Source: three-view drawing plus pictorial views. Frame: mm from the lowest corner of the part. A direction names the side the tool comes from. Give positions to 0.01 mm unless a question says otherwise; leave off trailing zeros. Order: outer loops, then holes, each group sorted by start corner. A loop starts at its lowest first (then second) coordinate and runs counter-clockwise, first axis right, second up. Notation, with made-up numbers: (-20.75, 38.25) -> (19.25, 38.25) arc R16 cw to (19.25, 65.25) -> close; hole circle Ø9 at (74.25, 35). An arc over 180 degrees is marked (long way). Use a Markdown table: item, result. Add a question column.
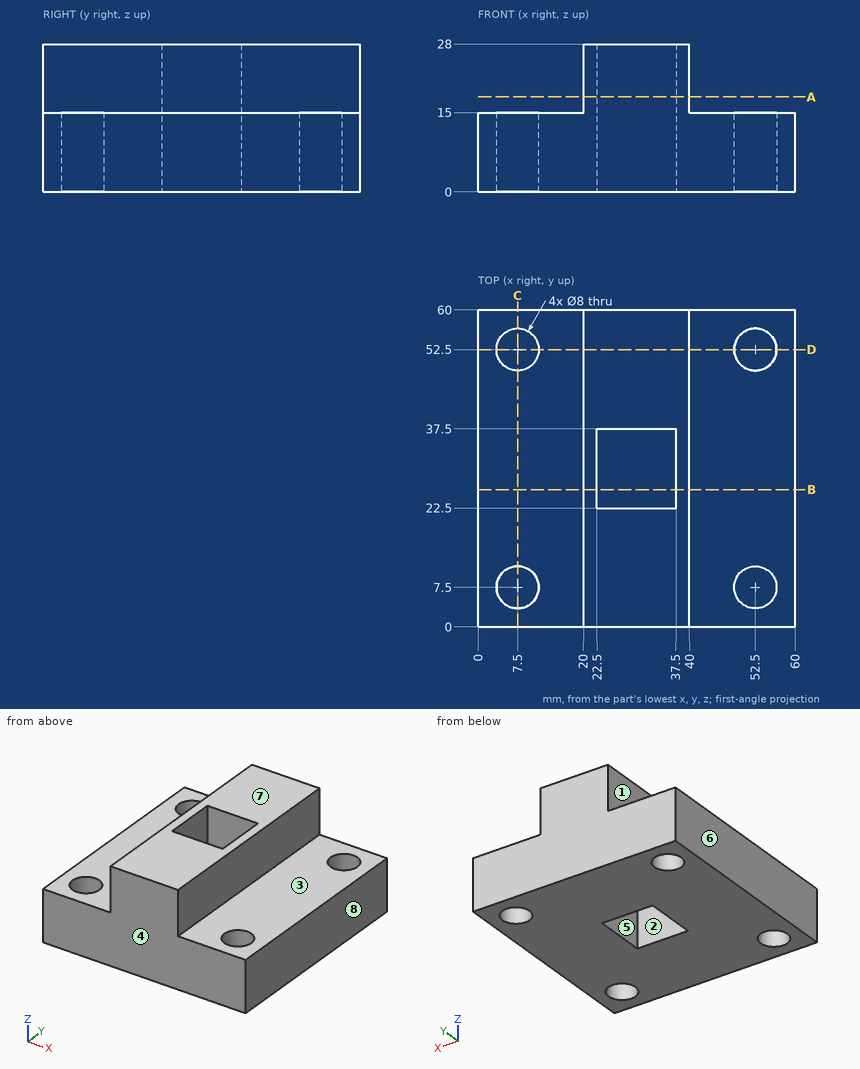
Q1. Section query A-A (z = 18). Return loops of the section in (x, y).
Q2. Access query for the marked faces 1, 2, 3 and 4. Directions: +Z, -Z, +X, -X, +Y, -Y. A direction counts if a zero-diameter tool reaches every point of the face in a straight line with its end or side. Return the directions, or none.
Q3. Section query C-C (x = 7.5). Return loops of the section in (y, z).
Q4. First-contact query: pin 1 (16 mm diameter, centred on x = 54.5, y = 19, fed in from +Z); pin 2 (6.5 mm diameter, centred on y = 31.5, z = 21, fed in from -X); pin 3 (6.5 mm diameter, centred on x = 7.5, y = 7.5, fed in from +Z). Flat tips, straight axial feed; report the tip coordinate or a pass-through.
Q5. Draft query along X for the marked faces 5, 6, 7 and 8. Return one class per face: +X half, -X half, draft (parallel to the pull), parting line (faces both ways), or undercut.
Q6. Ray query, line 1 (Y direction, x = 7.5, z = 4.75); line 2 (X direction, y = 26.5, z = 12); line 3 (Y direction, x = 54, z = 4). Return the intervals inside material, ascending.
Q7. Section query D-D (y = 52.5). Return loops of the section in (x, z), plus the area to 3 significant figures.
Q8. Section query B-B (y = 26). Return loops of the section in (x, z).
Solution:
| question | item | result |
|---|---|---|
| 1 | outline | (20, 0) -> (40, 0) -> (40, 60) -> (20, 60) -> close; hole (22.5, 22.5) -> (37.5, 22.5) -> (37.5, 37.5) -> (22.5, 37.5) -> close |
| 2 | face 1 | +Z, -X, +Y, -Y |
| 2 | face 2 | +Z, -Z |
| 2 | face 3 | +Z, +X, +Y, -Y |
| 2 | face 4 | +Z, -Z, +X, -X, -Y |
| 3 | outline | (0, 0) -> (3.5, 0) -> (3.5, 15) -> (0, 15) -> close; (11.5, 0) -> (48.5, 0) -> (48.5, 15) -> (11.5, 15) -> close; (56.5, 0) -> (60, 0) -> (60, 15) -> (56.5, 15) -> close |
| 4 | pin 1 | stops at z = 15 |
| 4 | pin 2 | stops at x = 20 |
| 4 | pin 3 | passes through |
| 5 | face 5 | undercut |
| 5 | face 6 | -X half |
| 5 | face 7 | draft |
| 5 | face 8 | +X half |
| 6 | line 1 | y = 0 to 3.5, 11.5 to 48.5, 56.5 to 60 |
| 6 | line 2 | x = 0 to 22.5, 37.5 to 60 |
| 6 | line 3 | y = 0 to 3.79, 11.21 to 48.79, 56.21 to 60 |
| 7 | outline | (0, 0) -> (3.5, 0) -> (3.5, 15) -> (0, 15) -> close; (11.5, 0) -> (48.5, 0) -> (48.5, 15) -> (40, 15) -> (40, 28) -> (20, 28) -> (20, 15) -> (11.5, 15) -> close; (56.5, 0) -> (60, 0) -> (60, 15) -> (56.5, 15) -> close |
| 7 | area | 920 mm² |
| 8 | outline | (0, 0) -> (22.5, 0) -> (22.5, 28) -> (20, 28) -> (20, 15) -> (0, 15) -> close; (37.5, 0) -> (60, 0) -> (60, 15) -> (40, 15) -> (40, 28) -> (37.5, 28) -> close |
